Input: part model. Units: mm. Frame: model coordinates. Face numbers are marked on the shaded views. A direction names the side the tool comes from. Give positions to 0.01 mm unless a question says otherwise; leave off trailing zeros. Write each loop counter-clockwise with the first axis right and the second up, starting at its lowest first coordinate (ties: lowest second). Pieces come first, ordered by that corner, then holes. Notation, with made-up numbers: (9, 20.25) -> (22, 20.25) arc R19 cw to (22, 52.25) -> close; hole circle Ø6 at (33.5, 80). An arc over 180 degrees is marked (long way). Return JSON: item names as keys, results as strings. Group by question number.
Item 1: Set-up query: the marked faces 5 and 6. Return all of +Z, -Z, +X, -X, +Y, -Y with unobstructed straight access to the full face (end or side cutting, diameter ignored); none if empty.
Item 2: Pin query (flat end, axial travel): P1, Ø4, axis at x = 3, y = -1.5, coming from the -Z side; P2, Ø12, axis at x = -1, y = -4.5, coming from the -Z side. Return the tip coordinate at first contact, or that it passes through.
Item 3: Line query: line 1 (Y direction, x = 0, z = 2); line 2 (Z direction, x = 1.25, y = 4.75). Output: solid intervals per line, ascending. Write a range as [from, to].
Item 4: Section B-B, the plane x = -5.5. Return loops of the section in (y, z).
Item 5: Section A-A, the plane y = 0. Return loops of the section in (x, z).
Item 6: Mould query, pull axis Y, two halves, no side actions, for the marked faces 1, 2, 3 and 4. Classes: released by +Y, released by -Y, zero draft, split by the parting line, or undercut.
from build123d import *

# Parameters (mm, degrees)
F0_W     = 25.4
F0_H     = 25.4
F1_DEPTH = 25.4
F2_R     = 6.35
F3_DEPTH = 6.35
F4_R     = 6.35
F5_DEPTH = 6.35


with BuildPart() as f1:
    # F0 (on Top) → F1 (new body)
    with BuildSketch(Plane.XY):
        Rectangle(F0_W, F0_H)
    extrude(amount=F1_DEPTH)

    # F2 (on face) → F3 (cut)
    with BuildSketch(Plane(origin=(0, 0, 0), x_dir=(1, 0, 0), z_dir=(0, 0, -1))):
        Circle(F2_R)
    extrude(amount=-F3_DEPTH, mode=Mode.SUBTRACT)

    # F4 (on face) → F5 (join)
    with BuildSketch(Plane.XY.offset(25.4)):
        Circle(F4_R)
    extrude(amount=F5_DEPTH)


solid = f1.part
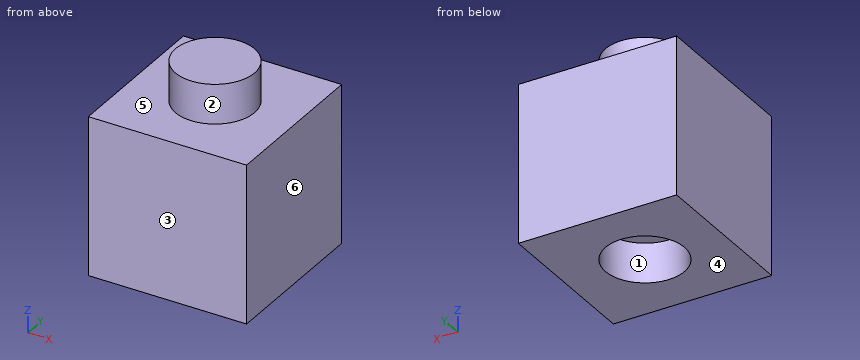
Answer below:
{
 "1": {"face 5": "+Z", "face 6": "+Z, -Z, +X, +Y, -Y"},
 "2": {"P1": "stops at z = 6.35", "P2": "stops at z = 0"},
 "3": {"line 1": "y = [-12.7, -6.35], [6.35, 12.7]", "line 2": "z = [6.35, 31.75]"},
 "4": {"outline": "(-12.7, 0) -> (-3.17, 0) -> (-3.17, 6.35) -> (3.17, 6.35) -> (3.17, 0) -> (12.7, 0) -> (12.7, 25.4) -> (3.17, 25.4) -> (3.17, 31.75) -> (-3.17, 31.75) -> (-3.17, 25.4) -> (-12.7, 25.4) -> close"},
 "5": {"outline": "(-12.7, 0) -> (-6.35, 0) -> (-6.35, 6.35) -> (6.35, 6.35) -> (6.35, 0) -> (12.7, 0) -> (12.7, 25.4) -> (6.35, 25.4) -> (6.35, 31.75) -> (-6.35, 31.75) -> (-6.35, 25.4) -> (-12.7, 25.4) -> close"},
 "6": {"face 1": "undercut", "face 2": "split by the parting line", "face 3": "released by -Y", "face 4": "zero draft"}
}
